Could you check a few things on this model? Use its own coordinates, in mm. A direction names the side the tool comes from. Give positions to 0.01 mm unless a question says otherwise; leave off trailing zeros. Loops run counter-clockwise (first coordinate to the right, second up) from the corner with the lowest first, then second, coordinate; pieces in that order, holes last. Notation, with made-up numbers: (40, 54) -> (82, 54) arc R15 ccw to (82, 61) -> close; hole circle Ø5 at (21.25, -22). An arc over 180 degrees is marked (long way). Put each result on its own line as item: value.
```python
from build123d import *

# Parameters (mm, degrees)
F0_W     = 5
F0_H     = 5
F1_DEPTH = 8
F2_R     = 1.5
F3_DEPTH = 25
F4_W     = 1
F4_H     = 8
F5_DEPTH = 47
F6_W     = 1
F6_H     = 8
F6_W_2   = 4
F7_DEPTH = 5
F8_R     = 1.5
F9_DEPTH = 25


with BuildPart() as f1:
    # F0 (on Top) → F1 (new body)
    with BuildSketch(Plane.XY):
        with Locations((2.5, 2.5)):
            Rectangle(F0_W, F0_H)
    extrude(amount=F1_DEPTH)

    # F2 (on face) → F3 (cut)
    with BuildSketch(Plane.XY.offset(8)):
        with Locations((2.5, 2.5)):
            Circle(F2_R)
    extrude(amount=-F3_DEPTH, mode=Mode.SUBTRACT)

    # F4 (on face) → F5 (join)
    with BuildSketch(Plane.XZ):
        with Locations((4.5, 4)):
            Rectangle(F4_W, F4_H)
    extrude(amount=F5_DEPTH)

    # F6 (on face) → F7 (join)
    with BuildSketch(Plane.XZ.offset(47)):
        with Locations((4.5, 4)):
            Rectangle(F6_W, F6_H)
        with Locations((2, 4)):
            Rectangle(F6_W_2, F6_H)
    extrude(amount=F7_DEPTH)

    # F8 (on face) → F9 (cut)
    with BuildSketch(Plane.XY.offset(8)):
        with Locations((2.5, -49.5)):
            Circle(F8_R)
    extrude(amount=-F9_DEPTH, mode=Mode.SUBTRACT)


solid = f1.part
```
1. If we section it at D-D (y = -12): List the corners of the cut face in (x, z) for me, then the cut area to 3 significant figures.
Recorded:
outline: (4, 0) -> (5, 0) -> (5, 8) -> (4, 8) -> close
area: 8.00 mm^2
2. If we section it at C-C (x = 2.55): List the corners of the cut face in (y, z) for me, then the cut area to 3 significant figures.
Recorded:
outline: (-52, 0) -> (-51, 0) -> (-51, 8) -> (-52, 8) -> close; (-48, 0) -> (-47, 0) -> (-47, 8) -> (-48, 8) -> close; (0, 0) -> (1, 0) -> (1, 8) -> (0, 8) -> close; (4, 0) -> (5, 0) -> (5, 8) -> (4, 8) -> close
area: 32.0 mm^2
3. Thinking about a two-plate mould opening in X: for faces 1 (the face through (2.175, -50.964, 4.056)), 2 (the face through (2, -52, 4)), 3 (the face through (4, -23, 4)), which applies, pulls with the +X half, pulls with the -X half, needs draft (parallel to the pull), parting line crosses it, or undercut?
Recorded:
face 1: undercut
face 2: needs draft
face 3: pulls with the -X half
4. If we section it at A-A (y = -49.5): List the corners of the cut face in (x, z) for me.
Recorded:
outline: (0, 0) -> (1, 0) -> (1, 8) -> (0, 8) -> close; (4, 0) -> (5, 0) -> (5, 8) -> (4, 8) -> close
5. I need wall thicknesses on line 1 (Y direction, x = 2.5, z = 5.25); line 2 (Y direction, x = 3.55, z = 6.75); line 3 (X direction, y = -42.5, z = 3). Which ranges of each line are inside material? Lowest first, please.
Recorded:
line 1: y = -52 to -51, -48 to -47, 0 to 1, 4 to 5
line 2: y = -52 to -50.57, -48.43 to -47, 0 to 1.43, 3.57 to 5
line 3: x = 4 to 5
6. For faces 4 (the face through (0, 2, 4)), 5 (the face through (2, 0, 4)), which set-ups out of +Z, -Z, +X, -X, +Y, -Y let a thin tool reach every point of the face, with its end or its side?
Recorded:
face 4: +Z, -Z, -X, +Y, -Y
face 5: +Z, -Z, -X
7. I'm going to push a flat-ended pin straight in: pin 1 (2.5 mm diameter, centred on y = -15.5, z = 4.5, fed in from -X). Where does the tip first touch, or does it pass through?
Recorded:
pin 1: stops at x = 4
8. If we section it at B-B (z = 2.5): List the corners of the cut face in (x, y) for me.
Recorded:
outline: (0, -52) -> (5, -52) -> (5, 5) -> (0, 5) -> (0, 0) -> (4, 0) -> (4, -47) -> (0, -47) -> close; hole circle Ø3 at (2.5, -49.5); hole circle Ø3 at (2.5, 2.5)
